For this review, take the finished solid that the model builds, in its own axes (mm). Give positions to 0.01 mm unless a question says otherwise; leave off trailing zeros. Loops run counter-clockwise (first coordinate to the right, second up) from the corner with the lowest first, then second, coordinate; pieces in that order, holes last. Notation, with made-up numbers: (66.5, 60.25) - (104.5, 60.25) arc R15 cw to (104.5, 84.25) - close; hole circle Ø1 at (86, 78). An arc over 180 degrees is marked (long way). Use CSV: the item, a comma, the result in double quotes. Start each with the question number.
1. Take a section at B-B on x = 27.5. Give the boundary of the cut face in (y, z), plus the area to 3 significant figures.
2. Wall thickness on line 1 (X direction, y = 6, z = 0); line 2 (X direction, y = 3.75, z = -3); line 3 (X direction, y = 3.5, z = -22): over which ranges is each line inside the solid? List them lowest first.
3. For pin 1 (4 mm diameter, centred on y = 6.5, z = -4.5, fed in from -X); pin 2 (4 mm diameter, centred on y = 5, z = -49, fed in from -X); pin 3 (4 mm diameter, centred on y = 6.5, z = -52, fed in from -X); pin 4 (2 mm diameter, centred on x = 0, z = 0, fed in from -Y), all flat-tipped, find the tip position at first contact; note any pin that passes through.
4. Take a section at A-A on y = 1.25. Give the boundary of the cut face in (x, z), plus the area to 3 significant figures.
5. Take a section at C-C on z = -19. Give the boundary of the cut face in (x, y), plus the area to 3 significant figures.
6. Take a section at D-D on x = 5.5. Give the boundary of the cut face in (y, z).
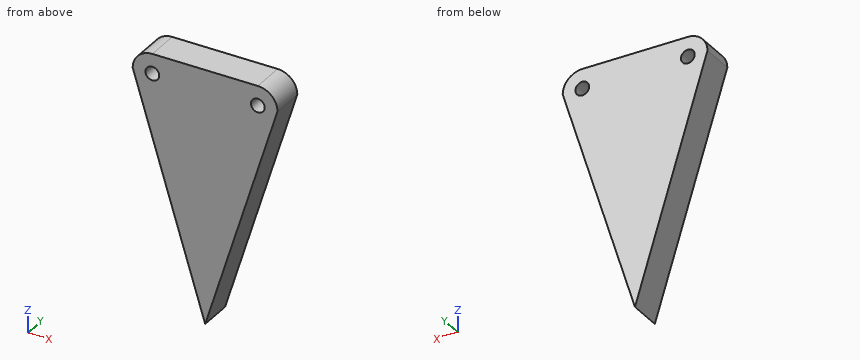
```python
from build123d import *

# Parameters (mm, degrees)
SKETCH1_R           = 1.75
BOSS_EXTRUDE3_DEPTH = 8.5


with BuildPart() as part:
    # Sketch1 → Boss-Extrude3 (new body)
    with BuildSketch(Plane(origin=(0, 0, 0), x_dir=(1, 0, 0), z_dir=(0, 1, 0))):
        with BuildLine():
            Line((-5, 0), (13.479806433, 59.697025207))
            Line((13.479806433, 59.697025207), (31.9, 0))
            ThreePointArc((31.9, 0), (30.435533906, -3.535533906), (26.9, -5))
            Line((26.9, -5), (0, -5))
            ThreePointArc((0, -5), (-3.535533906, -3.535533906), (-5, 0))
        make_face()
        with Locations(Location((0, 0, 0), (0, 0, 270))):
            Circle(SKETCH1_R, mode=Mode.SUBTRACT)
        with Locations(Location((26.9, 0, 0), (0, 0, 270))):
            Circle(SKETCH1_R, mode=Mode.SUBTRACT)
    extrude(amount=BOSS_EXTRUDE3_DEPTH)


solid = part.part
```
Check result:
1,outline,"(0, -14.26) - (8.5, -14.26) - (8.5, -1.64) - (0, -1.64) - close; (0, 1.64) - (8.5, 1.64) - (8.5, 4.96) - (0, 4.96) - close"
1,area,"135 mm²"
2,line 1,"x = -5 to -1.75, 1.75 to 25.15, 28.65 to 31.9"
2,line 2,"x = -4.07 to 30.97"
2,line 3,"x = 1.81 to 25.11"
3,pin 1,"stops at x = -4.23"
3,pin 2,"stops at x = 9.55"
3,pin 3,"stops at x = 10.48"
3,pin 4,"passes through"
4,outline,"(-5, 0) - (13.48, -59.7) - (31.9, 0) arc R5 ccw to (26.9, 5) - (0, 5) arc R5 ccw to start; hole circle Ø3.5 at (0, 0); hole circle Ø3.5 at (26.9, 0)"
4,area,"1,260 mm²"
5,outline,"(0.88, 0) - (26.04, 0) - (26.04, 8.5) - (0.88, 8.5) - close"
5,area,"214 mm²"
6,outline,"(0, -33.92) - (8.5, -33.92) - (8.5, 5) - (0, 5) - close"
